```python
from build123d import *

# Parameters (mm, degrees)
SKETCH_1_W          = 220
SKETCH_1_H          = 200
EXTRUDE_1_DEPTH     = 20
SKETCH_2_W          = 16
SKETCH_2_H          = 200
EXTRUDE_2_DEPTH     = 200
SKETCH_3_R          = 25
CUT_EXTRUDE_1_DEPTH = 295.319554226
SKETCH_4_W          = 8
SKETCH_4_H          = 80
EXTRUDE_3_DEPTH     = 52
CUT_EXTRUDE_2_DEPTH = 259.406656261
SKETCH_6_R          = 6
CUT_EXTRUDE_3_DEPTH = 16


with BuildPart() as part:
    # 草图1 → 凸台-拉伸1 (new body)
    with BuildSketch(Plane(origin=(0, 0, 0), x_dir=(1, 0, 0), z_dir=(0, 1, 0))):
        Rectangle(SKETCH_1_W, SKETCH_1_H)
    extrude(amount=EXTRUDE_1_DEPTH)

    # 草图2 → 凸台-拉伸2 (add)
    with BuildSketch(Plane(origin=(0, 20, 0), x_dir=(1, 0, 0), z_dir=(0, 1, 0))):
        with Locations((-50, 0)):
            Rectangle(SKETCH_2_W, SKETCH_2_H)
        with Locations((50, 0)):
            Rectangle(SKETCH_2_W, SKETCH_2_H)
    extrude(amount=EXTRUDE_2_DEPTH)

    # 草图3 → 切除-拉伸1 (cut, through all)
    with BuildSketch(Plane(origin=(58, 0, 0), x_dir=(0, 0, -1), z_dir=(1, 0, 0))):
        with Locations((0, 110)):
            Circle(SKETCH_3_R)
        with BuildLine():
            Line((-72.730270262, 128.311411403), (-100, 20))
            Line((-100, 20), (-100, 220))
            Line((-100, 220), (100, 220))
            Line((100, 220), (100, 20))
            Line((100, 20), (72.730270262, 128.311411403))
            ThreePointArc((72.730270262, 128.311411403), (0, 185), (-72.730270262, 128.311411403))
        make_face()
    extrude(amount=-CUT_EXTRUDE_1_DEPTH, mode=Mode.SUBTRACT)

    # 草图4 → 凸台-拉伸3 (add)
    with BuildSketch(Plane(origin=(58, 0, 0), x_dir=(0, 0, -1), z_dir=(1, 0, 0))):
        with Locations((-39, 60)):
            Rectangle(SKETCH_4_W, SKETCH_4_H)
        with Locations((39, 60)):
            Rectangle(SKETCH_4_W, SKETCH_4_H)
    extrude_3 = extrude(amount=EXTRUDE_3_DEPTH)

    # 草图5 → 切除-拉伸2 (cut, through all)
    with BuildSketch(Plane.XY.offset(43)):
        Polygon((110, 100), (78, 100), (110, 20), align=None)
    cut_extrude_2 = extrude(amount=-CUT_EXTRUDE_2_DEPTH, mode=Mode.SUBTRACT)

    # 镜向1: 凸台-拉伸3, 切除-拉伸2 across plane
    add(extrude_3.mirror(Plane(origin=(0, 0, 0), x_dir=(0, 0, 1), z_dir=(1, 0, 0))))
    add(cut_extrude_2.mirror(Plane(origin=(0, 0, 0), x_dir=(0, 0, 1), z_dir=(1, 0, 0))), mode=Mode.SUBTRACT)

    # 草图6 → 切除-拉伸3 (cut)
    with BuildSketch(Plane(origin=(58, 0, 0), x_dir=(0, 0, -1), z_dir=(1, 0, 0))):
        with Locations((-30, 143)):
            Circle(SKETCH_6_R)
        with Locations((30, 143)):
            Circle(SKETCH_6_R)
    extrude(amount=-CUT_EXTRUDE_3_DEPTH, mode=Mode.SUBTRACT)


solid = part.part
```
Input: part model. Units: mm. Frame: model coordinates. A direction names the side the tool comes from. Give positions to 0.01 mm unless a question says otherwise; leave off trailing zeros. Write each loop counter-clockwise with the first axis right and the second up, starting at its lowest first coordinate (ties: lowest second). Pieces come first, ordered by that corner, then holes. Notation, with made-up numbers: (-19, 6.25) - (2, 6.25) arc R12 ccw to (2, 17.25) - close; hole circle Ø5 at (-37, -6). An arc over 180 degrees is marked (long way). Write item = value, one per line. Start each with the question number.
1. Section query C-C, the plane z = 30. Output: boundary loops of the cut face in (x, y).
2. Access query for faces 1 (the flat face through (-68, 100, -39)), 2 (the flat face through (-84, 20, 71)), 3 (the flat face through (42, 83, 1)), 4 (the flat face through (68, 100, -39)). Directions: +Z, -Z, +X, -X, +Y, -Y. A direction counts if a zero-diameter tool reaches every point of the face in a straight line with its end or side. Return the directions, or none.
3. First-contact query: pin 1 Ø4 at (y, z) = (123, -24) entering from -X; pin 2 Ø6 at (x, y) = (-62.5, 137.5) entering from +Z; pin 3 Ø9 at (x, z) = (-71.5, -41) entering from +Y; pin 4 Ø10 at (x, z) = (76, 26.5) entering from +Y. Flat tips, straight axial feed; report the tip coordinate or a pass-through.
4. Mould query, pull axis Z, two halves, no side actions, for faces 5 (the flat face through (-78, 51, 35)), 6 (the flat face through (84, 20, 71)), 7 (the flat face through (50.112, 74.914, 86.174)), 8 (the flat face through (-78, 51, -35)). Classes: released by +Z, released by -Z, zero draft, split by the parting line, or undercut.
5. Section query B-B, the plane y = 93.5. Count the separate pieces of the cut face and the enclosed holes in it, then the cut area to 3 significant figures.
6. Section query A-A, the plane z = 0. Output: boundary loops of the cut face in (x, y).
7. Ray query, L1, parallel to X at y = 21.5, z = 84; L2, parallel to Z at x = 58.5, y = 24.5; L3, parallel to Y at x = 37.5, z = -44.5. Return the intervals inside material, ascending.
8. Section query D-D, the plane y = 34. Output: boundary loops of the cut face in (x, z), then the cut area to 3 significant figures.
Check sheet entries:
q1.outline = (-110, 0) - (110, 0) - (110, 20) - (58, 20) - (58, 137) - (42, 137) - (42, 20) - (-42, 20) - (-42, 178.74) - (-58, 178.74) - (-58, 20) - (-110, 20) - close; (42, 149) - (58, 149) - (58, 178.74) - (42, 178.74) - close
q2.face_1 = +Z, -Z, -X, +Y
q2.face_2 = +Z, -X, +Y
q2.face_3 = +Z, -Z, +Y
q2.face_4 = +Z, -Z, +X, +Y
q3.pin_1 = -58
q3.pin_2 = through
q3.pin_3 = 100
q3.pin_4 = 20
q4.face_5 = undercut
q4.face_6 = zero draft
q4.face_7 = released by +Z
q4.face_8 = undercut
q5.separate_pieces = 4
q5.enclosed_holes = 0
q5.area = 4,740 mm2
q6.outline = (-110, 0) - (110, 0) - (110, 20) - (58, 20) - (58, 85) - (42, 85) - (42, 20) - (-42, 20) - (-42, 85) - (-58, 85) - (-58, 20) - (-110, 20) - close; (-58, 135) - (-42, 135) - (-42, 185) - (-58, 185) - close; (42, 135) - (58, 135) - (58, 185) - (42, 185) - close
q7.L1 = -58 to -42, 42 to 58
q7.L2 = -43 to -35, 35 to 43
q7.L3 = 0 to 20
q8.outline = (-104.4, -43) - (-58, -43) - (-58, -96.48) - (-42, -96.48) - (-42, 96.48) - (-58, 96.48) - (-58, 43) - (-104.4, 43) - (-104.4, 35) - (-58, 35) - (-58, -35) - (-104.4, -35) - close; (42, -96.48) - (58, -96.48) - (58, -43) - (104.4, -43) - (104.4, -35) - (58, -35) - (58, 35) - (104.4, 35) - (104.4, 43) - (58, 43) - (58, 96.48) - (42, 96.48) - close
q8.area = 7,660 mm2
